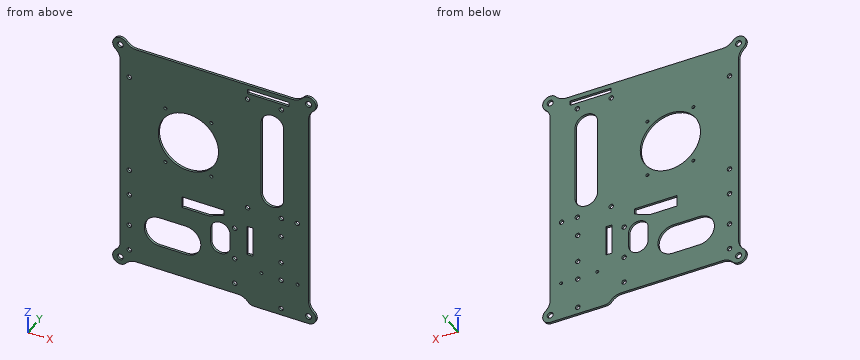
Autodesk Fusion 360 part; units mm, degrees
sketch "Sketch1" plane through (0, 0, 0) normal (0, 1, 0) x (1, 0, 0)
  arc A0 (25.8589, 127) -> (18.199, 123.4286) centre (25.8589, 117) ccw
  circle A1 centre (62, 16) radius 3
  arc A2 (4.4113, 117) -> (18.199, 123.4286) centre (4.4113, 135) ccw
  line L0 (-64.5, 44) -> (-99.5, 44)
  line L1 (-151.5, 95.5524) -> (-151.5, -162.5524)
  line L2 (98.5, -162.5524) -> (98.5, 95.5524)
  line L3 (-31.5, 36) -> (-31.5, 54)
  circle A3 centre (-151.5, -184) radius 4
  arc A4 (-130.0524, -184) -> (-143.8401, -190.4286) centre (-130.0524, -202) ccw
  line L4 (-13.5, 4) -> (-69.5, 4)
  line L5 (-69.5, 19) -> (-13.5, 19)
  line L6 (-69.5, 4) -> (-69.5, 19)
  circle A5 centre (62.5, -10) radius 3
  line L7 (-130.0524, -184) -> (77.0524, -184)
  circle A6 centre (83.5, -10) radius 3
  line L8 (4.4113, 117) -> (-130.0524, 117)
  circle A7 centre (0.5, 103) radius 3
  circle A8 centre (62, 53) radius 3
  arc A9 (-157.9286, -176.3401) -> (-143.8401, -190.4286) centre (-151.5, -184) ccw
  arc A10 (-151.5, 95.5524) -> (-157.9286, 109.3401) centre (-169.5, 95.5524) ccw
  arc A11 (104.9286, 109.3401) -> (98.5, 127) centre (98.5, 117) ccw
  circle A12 centre (-139.5, 103) radius 3
  arc A13 (104.9286, 109.3401) -> (98.5, 95.5524) centre (116.5, 95.5524) ccw
  arc A14 (-5.5, 54) -> (-31.5, 54) centre (-18.5, 54) ccw
  circle A15 centre (0.5, 25) radius 3
  arc A16 (-31.5, 36) -> (-5.5, 36) centre (-18.5, 36) ccw
  circle A17 centre (98.5, 117) radius 4
  circle A18 centre (17.5, -10) radius 3
  circle A19 centre (-151.5, 117) radius 4
  circle A20 centre (-139.5, 25) radius 3
  circle A21 centre (62.5, -164) radius 3
  arc A22 (-157.9286, -176.3401) -> (-151.5, -162.5524) centre (-169.5, -162.5524) ccw
  arc A23 (98.5, -162.5524) -> (104.9286, -176.3401) centre (116.5, -162.5524) ccw
  arc A24 (65.5, -37) -> (35.5, -37) centre (50.5, -37) ccw
  line L9 (65.5, -37) -> (65.5, -137)
  line L10 (35.5, -137) -> (35.5, -37)
  arc A25 (35.5, -137) -> (65.5, -137) centre (50.5, -137) ccw
  circle A26 centre (98.5, -184) radius 4
  circle A27 centre (-30.5, -114) radius 2
  circle A28 centre (17.5, -164) radius 3
  circle A29 centre (-91.5, -114) radius 2
  arc A30 (90.8401, -190.4286) -> (77.0524, -184) centre (77.0524, -202) ccw
  arc A31 (90.8401, -190.4286) -> (104.9286, -176.3401) centre (98.5, -184) ccw
  circle A32 centre (-61, -76) radius 40
  circle A33 centre (-30.5, -38) radius 2
  circle A34 centre (-91.5, -38) radius 2
  circle A35 centre (-139.5, -142) radius 3
  circle A36 centre (62, 118) radius 3
  arc A37 (-64.5, 44) -> (-64.5, 84) centre (-64.5, 64) ccw
  line L11 (16.5, 56.5) -> (24.5, 56.5)
  circle A38 centre (-139.5, -10) radius 3
  line L12 (16.5, 16.5) -> (16.5, 56.5)
  line L13 (98.5, 127) -> (25.8589, 127)
  line L14 (-99.5, 84) -> (-64.5, 84)
  line L15 (-13.5, 19) -> (-13.5, 4)
  arc A39 (-143.8401, 123.4286) -> (-157.9286, 109.3401) centre (-151.5, 117) ccw
  arc A40 (-143.8401, 123.4286) -> (-130.0524, 117) centre (-130.0524, 135) ccw
  arc A41 (-99.5, 84) -> (-99.5, 44) centre (-99.5, 64) ccw
  line L16 (24.5, 56.5) -> (24.5, 16.5)
  line L17 (-5.5, 54) -> (-5.5, 36)
  line L18 (24.5, 16.5) -> (16.5, 16.5)
  line L19 (-34.0405, 19) -> (-13.5, 11.5)
  line L20 (62.5, -164) -> (72.5, -164) construction
  line L21 (72.5, -164) -> (72.5, -172) construction
  line L22 (72.5, -172) -> (62.5, -172) construction
  line L23 (62.5, -172) -> (62.5, -164) construction
  line L24 (17.5, -164) -> (17.5, -172) construction
  line L25 (17.5, -172) -> (72.5, -172)
  line L26 (72.5, -172) -> (72.5, -178.01)
  line L27 (72.5, -178.01) -> (17.5, -178.01)
  line L28 (17.5, -178.01) -> (17.5, -172)
  circle A42 centre (36, 76.5) radius 2
  circle A43 centre (84, 76.5) radius 2
  circle A44 centre (-139.5, 68) radius 3
  circle A45 centre (0.5, 68) radius 3
  circle A46 centre (62, 78) radius 3
  point P0 (-61, -76)
  dimension "d5" = 10
  dimension "d6" = 8
  dimension "d7" = 8
  dimension "d8" = 6.01
  dimension "d9" = 4
  dimension "d10" = 48
extrude "Extrude1" add sketch "Sketch1" along normal blind 3 contours A0 A2 L1 L2 A4 L7 L8 A9 A10 A11 A13 A22 A23 A30 A31 L13 A39 A40 | L5 L15 L19
equation "d7 = d6"
Read the model definition and answer for the solid it produces. Units are mm, in the model's axes. Coordinates: 2 decimals unless noted, no trailing zeros. Loops run counter-clockwise (first coordinate to the right, second up) from the corner with the lowest first, then second, coordinate; pieces in that order, holes last.
(1) Consider line 1 along X through (y, z) = (2.1, 164); line 2 along Z through (x, y) = (1, 0.3); line 3 along X through (y, z) = (2.4, 73.5). Determine where each line is inside the solid, lowest interval first.
Solution:
line 1: x = -151.56 to 14.5, 20.5 to 59.5, 65.5 to 98.56
line 2: z = -117 to -105.96, -100.04 to -70.96, -65.04 to -27.96, -22.04 to 184
line 3: x = -151.5 to -100.92, -21.08 to 35.5, 65.5 to 98.5
(2) The part is cut by section C-C (y = 1.25). Count the separate pieces of the cut face and the enclosed holes in it, and give its area (3 significant figures).
Solution:
separate pieces: 1
enclosed holes: 34
area: 62,500 mm2
(3) Flat-ended cylindrical pins translate along their axes: pin 1 Ø1.5 at (y, z) = (2, 174) entering from +X; pin 2 Ø1.5 at (y, z) = (1, -39) entering from +X; pin 3 Ø0.9 at (x, y) = (19.5, 2) entering from +Z. Find the tip coordinate at first contact, or state that the pin passes through.
Solution:
pin 1: stops at x = 103.26
pin 2: stops at x = 98.5
pin 3: stops at z = 184
(4) The part is cut by section B-B (x = -106). Determine the outline of the cut face in (y, z).
Solution:
outline: (0, -117) - (3, -117) - (3, -82.91) - (0, -82.91) - close; (0, -45.09) - (3, -45.09) - (3, 184) - (0, 184) - close
(5) The part is cut by section D-D (x = 49.5). Determine the outline of the cut face in (y, z), and give its area (3 significant figures).
Solution:
outline: (0, -127) - (3, -127) - (3, 22.03) - (0, 22.03) - close; (0, 151.97) - (3, 151.97) - (3, 172) - (0, 172) - close; (0, 178.01) - (3, 178.01) - (3, 184) - (0, 184) - close
area: 525 mm2
(6) The part is cut by section A-A (x = -61). Determine the outline of the cut face in (y, z), and give its area (3 significant figures).
Solution:
outline: (0, -117) - (3, -117) - (3, -83.69) - (0, -83.69) - close; (0, -44.31) - (3, -44.31) - (3, -19) - (0, -19) - close; (0, -4) - (3, -4) - (3, 36) - (0, 36) - close; (0, 116) - (3, 116) - (3, 184) - (0, 184) - close
area: 500 mm2
